Model file for the job. Use its own axes, mm. A direction names the side the tool comes from. Give positions to 0.01 mm unless a question says otherwise; leave off trailing zeros. Loops run counter-clockwise (first coordinate to the right, second up) from the corner with the lowest first, then second, coordinate; pieces in that order, holes last. Notation, with made-up numbers: (62.25, 53) - (116.25, 53) arc R25 cw to (116.25, 77) - close; hole circle Ø6 at (-39, -6). An arc over 180 degrees is marked (long way). Answer as CSV lines item,"result". Start each with the question number.
Item 1: Saw through at A-A on x = -25.5. Give the cut face in (y, z), plus the area to 3 significant figures.
Item 2: Saw through at D-D on z = -9.5. Give the cut face in (x, y), plus the area to 3 significant figures.
Item 3: Tool access for faces 5 (the flat face through (0, 17, 2)), 6 (the cylindrical face through (-49, 2, -57)), 7 (the flat face through (5, 2, -93)), 8 (the flat face through (-23, 22.5, 3)), 9 (the flat face through (-13, 3, -61)): list every direction of +Z, -Z, +X, -X, +Y, -Y with a clear straight run to the whole face (end or side of a thin tool).
Item 4: Saw through at B-B on y = 17.5. Give the cut face in (x, z), plus the area to 3 significant figures.
Item 5: Drill centre lines: L1, parallel to Z at x = -27, y = 11.25; L2, parallel to Y at x = -13, z = -37; L3, parallel to X at y = 22.75, z = -70. Where is each one in solid material? Low to high. Write a range as from..to.
Item 6: Pull direction Z, two halves, no side cores. Call faces 1 (the flat face through (-20, 0, -57)), 2 (the cylindrical face through (-7, 2, -90)), 3 (the flat face through (-12, 3, -91)), 4 (the cylindrical face through (-20, 2, 4)): pulls with the +Z half, pulls with the -Z half, needs draft (parallel to the pull), parting line crosses it, or undercut.
Item 7: Pin check, flat tips, straight feed: pin 1 (1 mm diameter, centred on x = -28, z = -92, fed in from +Y); pin 2 (1.5 mm diameter, centred on x = -12, y = 2, fed in from +Z); pin 3 (1.5 mm diameter, centred on x = -13, y = 3.5, fed in from -Z). Stop position of each tip, or through.
Item 8: Saw through at C-C on x = -7.5. Give the cut face in (y, z), plus the area to 3 significant figures.
Autodesk Inventor part; units mm, degrees
ref_plane "YZ Plane" through (0, 0, 0) normal (1, 0, 0) x (0, 1, 0)
ref_plane "XZ Plane" through (0, 0, 0) normal (0, 1, 0) x (-1, 0, 0)
ref_plane "XY Plane" through (0, 0, 0) normal (0, 0, 1) x (1, 0, 0)
sketch "Sketch1" plane through (0, 0, 0) normal (0, 1, 0) x (-1, 0, 0)
  line L0 (0, 0) -> (45, 0)
  line L1 (45, 0) -> (45, -115)
  line L2 (45, -115) -> (0, -115)
  line L3 (0, -115) -> (0, 0)
  line L4 (50, -120) -> (50, 5)
  line L5 (50, 5) -> (-5, 5)
  line L6 (-5, 5) -> (-5, -120)
  line L7 (-5, -120) -> (50, -120)
  dimension "d0" = 45
  dimension "d1" = 115
  dimension "d2" = 5
extrude "Extrusion1" add sketch "Sketch1" along normal blind 5 contours L0 L1 L2 L3 | L7 L6 L5 L4
sketch "Sketch2" plane through (0, 5, 0) normal (0, 1, 0) x (1, 0, 0)
  line L0 (0, 0) -> (-45, 0)
  line L1 (-45, 0) -> (-45, 115)
  line L2 (-45, 115) -> (0, 115)
  line L3 (0, 115) -> (0, 0)
  line L4 (5, 120) -> (-50, 120)
  line L5 (-50, 120) -> (-50, -5)
  line L6 (-50, -5) -> (5, -5)
  line L7 (0, 115) -> (0, 120)
  line L8 (5, 120) -> (-50, 120)
  line L9 (0, 0) -> (0, -5)
  dimension "d5" = 45
  dimension "d6" = 115
  dimension "d7" = 5
extrude "Extrusion2" add sketch "Sketch2" along normal blind 25 contours L9 L6 L5 L4 L7 L2 L1 L0
sketch "Sketch3" plane through (-50, 0, 5) normal (0, 0, 1) x (1, 0, 0)
  line L0 (5, 30) -> (50, 30)
  line L1 (27.5, 30) -> (27.5, 24.5)
  line L2 (17.5, 24.5) -> (37.5, 24.5) construction
  line L3 (17.5, 22.5) -> (37.5, 22.5)
  line L4 (37.5, 26.5) -> (17.5, 26.5)
  arc A0 (17.5, 26.5) -> (17.5, 22.5) centre (17.5, 24.5) ccw
  arc A1 (37.5, 22.5) -> (37.5, 26.5) centre (37.5, 24.5) ccw
  line L5 (27.5, 24.5) -> (47.5, 24.5) construction
  point P0 (50, 0)
  dimension "d10" = 5.5
  dimension "d11" = 10
  dimension "d12" = 0
  dimension "d13" = 4
extrude "Extrusion3" cut sketch "Sketch3" against normal blind 125
sketch "Sketch4" plane through (0, 5, 0) normal (0, 1, 0) x (1, 0, 0)
  line L0 (-45, 0) -> (-45, 115)
  line L1 (-45, 0) -> (-20, 0)
  line L2 (-45, 0) -> (0, 0)
  line L3 (-20, 0) -> (-20, 6)
  line L4 (-20, 6) -> (-5, 6)
  line L5 (-5, 6) -> (-5, 36)
  line L6 (-5, 36) -> (-20, 36)
  line L7 (-20, 36) -> (-20, 6)
  line L8 (-5, 91) -> (-20, 91)
  line L9 (-5, 61) -> (-5, 91)
  line L10 (-20, 91) -> (-20, 61)
  line L11 (-20, 61) -> (-5, 61)
  dimension "d16" = 25
  dimension "d17" = 6
  dimension "d18" = 15
  dimension "d19" = 30
  dimension "d22" = 55
extrude "Extrusion4" cut sketch "Sketch4" against normal blind 5
fillet "Fillet1" radius 5 5 edges at (-22.5, 0, 5) (-22.5, 0, -120) (-50, 0, -57.5) (-50, 15, 5) (-50, 15, -120)
fillet "Fillet2" radius 5 8 edges at (-20, 2.5, -6) (-5, 2.5, -36) (-5, 2.5, -91) (-20, 2.5, -36) (-20, 2.5, -91) (-5, 2.5, -6) (-5, 2.5, -61) (-20, 2.5, -61)
pattern_linear "Rectangular Pattern1" count 2 spacing 7 along (0, -1, 0) of "Extrusion3"
sketch "Sketch5" plane through (5, 0, 0) normal (1, 0, 0) x (0, 0, -1)
  line L0 (61, 0) -> (61, 5)
  line L1 (0, 0) -> (61, 0)
  line L2 (61, 0) -> (61, 5)
  line L3 (61, 5) -> (66, 5)
  line L4 (66, 5) -> (66, 0)
  line L5 (66, 0) -> (61, 0)
  line L6 (61, 5) -> (61, 0)
  line L7 (61, 0) -> (56, 0)
  line L8 (56, 0) -> (56, 5)
  line L9 (56, 5) -> (61, 5)
  dimension "d34" = 5
  dimension "d35" = 5
extrude "Extrusion5" cut sketch "Sketch5" against normal blind 3
properties part number "Power_Supply_Shroud"
Responses:
1,outline,"(0, -115) arc R5 ccw to (5, -120) - (15.5, -120) - (15.5, -115) - (5, -115) - (5, 0) - (15.5, 0) - (15.5, 5) - (5, 5) arc R5 ccw to (0, 0) - close; (19.5, -120) - (22.5, -120) - (22.5, -115) - (19.5, -115) - close; (19.5, 0) - (22.5, 0) - (22.5, 5) - (19.5, 5) - close; (26.5, -120) - (30, -120) - (30, -115) - (26.5, -115) - close; (26.5, 0) - (30, 0) - (30, 5) - (26.5, 5) - close"
1,area,"784 mm2"
2,outline,"(-50, 5) arc R5 ccw to (-45, 0) - (-19.77, 0) - (-19.77, 5) - (-45, 5) - (-45, 30) - (-50, 30) - close; (-5.23, 0) - (5, 0) - (5, 5) - (-5.23, 5) - close"
2,area,"322 mm2"
3,face 5,"+Z, -Z, +X, +Y"
3,face 6,"+Z, -Z, -X, -Y"
3,face 7,"+Z, -Z, +X, +Y, -Y"
3,face 8,"+Z, -Z"
3,face 9,"+Y, -Y"
4,outline,"(-50, -115) arc R5 ccw to (-45, -120) - (-34.5, -120) - (-34.5, -115) - (-45, -115) - (-45, 0) - (-34.5, 0) - (-34.5, 5) - (-45, 5) arc R5 ccw to (-50, 0) - close; (-10.5, -120) - (0, -120) - (0, -115) - (-10.5, -115) - close; (-10.5, 0) - (0, 0) - (0, 5) - (-10.5, 5) - close"
4,area,"824 mm2"
5,L1,"-120..-115, 0..5"
5,L2,"0..5"
5,L3,"-50..-45"
6,face 1,"needs draft"
6,face 2,"undercut"
6,face 3,"undercut"
6,face 4,"pulls with the +Z half"
7,pin 1,"y = 5"
7,pin 2,"z = 4.47"
7,pin 3,"z = -119.94"
8,outline,"(0, -115) arc R5 ccw to (5, -120) - (30, -120) - (30, -115) - (5, -115) - (5, -90.33) - (0, -90.33) - close; (0, -61.67) - (5, -61.67) - (5, -35.33) - (0, -35.33) - close; (0, -6.67) - (5, -6.67) - (5, 0) - (30, 0) - (30, 5) - (5, 5) arc R5 ccw to (0, 0) - close"
8,area,"578 mm2"
